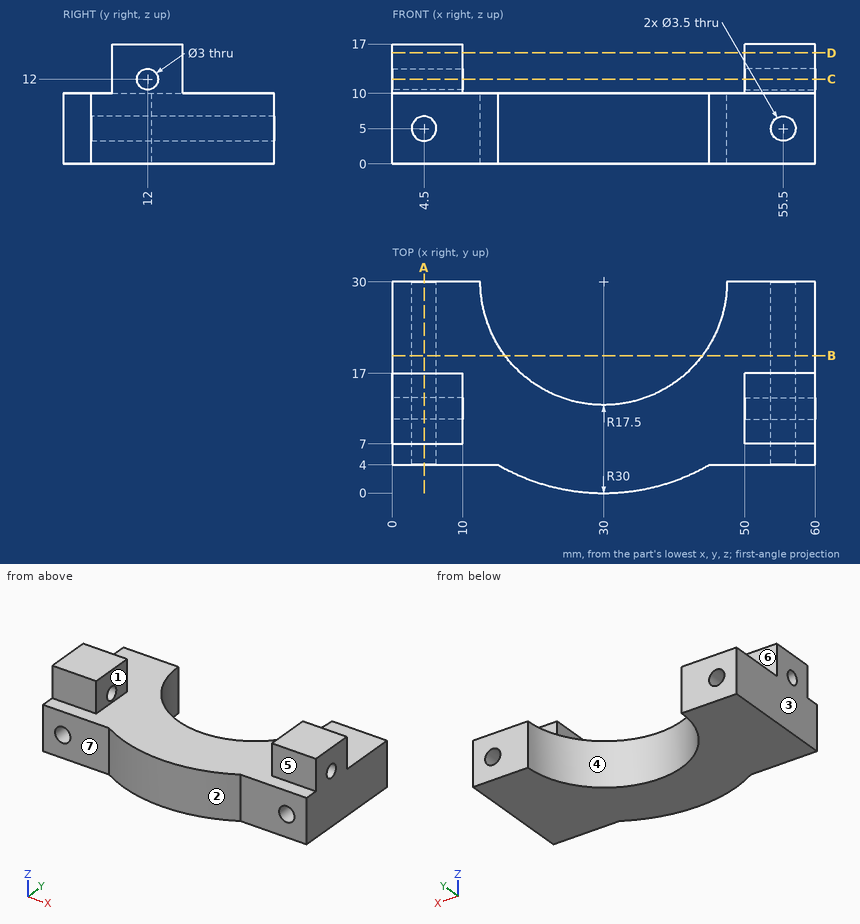
Geometry: see drawing. Coordinates: mm, zero at the bounding-box minimum. A direction names the side the tool comes from. Round coordinates to 2 decimals unless told otherwise and drop trailing zeros. Write each loop counter-clockwise with the first axis right and the second up, starting at its lowest first coordinate (ties: lowest second). Pieces come first, ordered by that corner, then holes.
Item 1: Section query A-A (x = 4.5). Return loops of the section in (y, z).
Item 2: Section query B-B (y = 19.5). Return loops of the section in (x, z).
Item 3: Mould query, pull axis X, two halves, no side actions, for the marked faces 1, 2, 3 and 4. Classes: +X half, -X half, draft (parallel to the pull), parting line (faces both ways), or undercut.
Item 4: Set-up query: the marked faces 5, 6 and 7. Return all of +Z, -Z, +X, -X, +Y, -Y with unobstructed straight access to the full face (end or side cutting, diameter ignored); none if empty.
Item 5: Pin query (flat end, axial travel): P1, Ø8, axis at x = 10, z = 4, coming from the -Y side; P2, Ø4, axis at x = 19.5, z = 7, coming from the -Y side; P3, Ø2, axis at x = 6.5, z = 13, coming from the +Y side. Return the tip coordinate at first contact, or that it passes through.
Item 6: Section query C-C (z = 12). Return loops of the section in (x, y), plus the area to 3 significant figures.
Item 7: Section query D-D (z = 15.75). Return loops of the section in (x, y).
Item 8: Material intervals for L1, parallel to X at y = 11.25, z = 5; L2, parallel to X at y = 9.5, z = 3.75; L3, parallel to Z at x = 4.5, y = 15, sorted ascending.
Completed:
1. outline: (4, 0) - (30, 0) - (30, 3.25) - (4, 3.25) - close; (4, 6.75) - (30, 6.75) - (30, 10) - (17, 10) - (17, 17) - (7, 17) - (7, 10) - (4, 10) - close; hole circle Ø3 at (12, 12)
2. outline: (0, 0) - (16, 0) - (16, 10) - (0, 10) - close; (44, 0) - (60, 0) - (60, 10) - (44, 10) - close; hole circle Ø3.5 at (4.5, 5); hole circle Ø3.5 at (55.5, 5)
3. face 1: undercut
3. face 2: parting line
3. face 3: -X half
3. face 4: undercut
4. face 5: +Z, +X, -X, -Y
4. face 6: +Z, +X, -X, +Y
4. face 7: +Z, -Z, -X, -Y
5. P1: stops at y = 4
5. P2: stops at y = 1.23
5. P3: stops at y = 17
6. outline: (0, 7) - (10, 7) - (10, 10.5) - (0, 10.5) - close; (0, 13.5) - (10, 13.5) - (10, 17) - (0, 17) - close; (50, 7) - (60, 7) - (60, 10.5) - (50, 10.5) - close; (50, 13.5) - (60, 13.5) - (60, 17) - (50, 17) - close
6. area: 140 mm2
7. outline: (0, 7) - (10, 7) - (10, 17) - (0, 17) - close; (50, 7) - (60, 7) - (60, 17) - (50, 17) - close
8. L1: x = 0 to 2.75, 6.25 to 53.75, 57.25 to 60
8. L2: x = 0 to 3.28, 5.72 to 54.28, 56.72 to 60
8. L3: z = 0 to 3.25, 6.75 to 17
